Study the drawing (mm; zero at the part's minimum x, y, z) and answer. A direction names the side the tool comes from. Round coordinates to 2 decimals unless told otherwise and drop trailing zeros. Write each loop counter-clockwise with the first axis right and the second up, starting at its lowest first coordinate (ties: lowest second). Pieces come first, ordered by that corner, then holes. Notation, with made-up numbers: (33, 59.25) -> (47, 59.25) arc R19 cw to (47, 69.25) -> close; hole circle Ø3 at (29, 33). An arc over 180 degrees is marked (long way). Return JSON: item names as keys, results as strings.
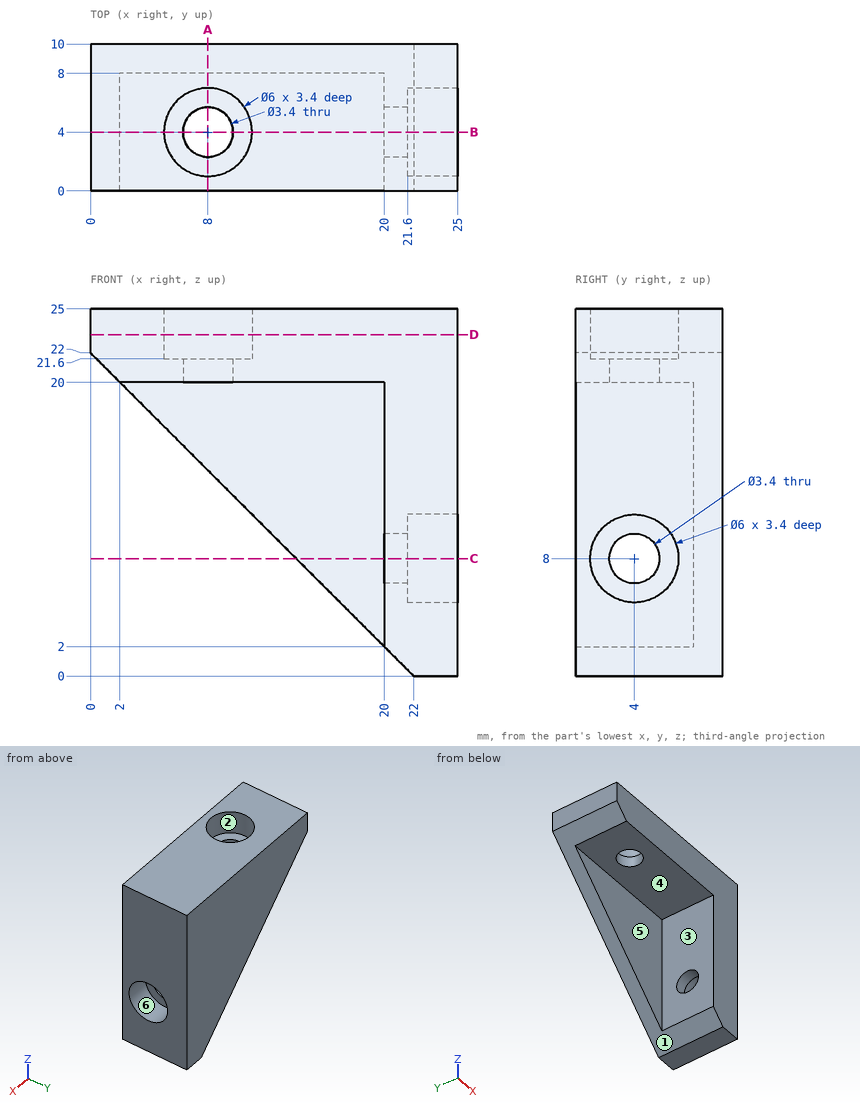
Item 1: Section D-D (z = 23.25) is taken. Give the vertices of the cut face in (x, y).
Worked answers:
{"outline": "(0, 0) -> (25, 0) -> (25, 10) -> (0, 10) -> close; hole circle Ø6 at (8, 4)"}
Item 2: Flat-ended cylindrical pins translate along their axes: pin 1 (5 mm diameter, centred on x = 8, y = 4, fed in from -Z); pin 2 (5 mm diameter, centred on x = 14, z = 3, fed in from -Y); pin 3 (6 mm diameter, centred on y = 3, z = 10.5, fed in from -X); pin 4 (1.8 mm diameter, centred on y = 4.5, z = 9.5, fed in from +X). Find the tip coordinate at first contact, or state that the pin passes through.
Worked answers:
{"pin 1": "stops at z = 20", "pin 2": "passes through", "pin 3": "stops at x = 20", "pin 4": "stops at x = 21.6"}
Item 3: Section A-A (x = 8) is taken. Give the vertices of the cut face in (y, z), then the cut area to 3 significant figures.
Worked answers:
{"outline": "(0, 20) -> (2.3, 20) -> (2.3, 21.6) -> (1, 21.6) -> (1, 25) -> (0, 25) -> close; (5.7, 20) -> (8, 20) -> (8, 14) -> (10, 14) -> (10, 25) -> (7, 25) -> (7, 21.6) -> (5.7, 21.6) -> close", "area": "36.2 mm2"}
Item 4: For a pull along Y with two mould halves and no side action, classify the marked faces 4, 5 and 6 as released by +Y, released by -Y, zero draft, split by the parting line, or undercut.
Worked answers:
{"face 4": "zero draft", "face 5": "released by -Y", "face 6": "undercut"}
Item 5: Straight lines are drawn through the part: L1, parallel to Y at x = 8, z = 22.8; L2, parallel to Y at x = 21.15, z = 8; L3, parallel to Z at x = 23.25, y = 4. For each, find the intervals that lie inside material, in ascending order. Write a range as [from, to].
Worked answers:
{"L1": "y = [0, 1], [7, 10]", "L2": "y = [0, 2.3], [5.7, 10]", "L3": "z = [0, 5], [11, 25]"}
Item 6: Section C-C (z = 8) is taken. Give the vertices of the cut face in (x, y), then the cut area to 3 significant figures.
Worked answers:
{"outline": "(14, 8) -> (20, 8) -> (20, 5.7) -> (21.6, 5.7) -> (21.6, 7) -> (25, 7) -> (25, 10) -> (14, 10) -> close; (20, 0) -> (25, 0) -> (25, 1) -> (21.6, 1) -> (21.6, 2.3) -> (20, 2.3) -> close", "area": "36.2 mm2"}
Item 7: A tool of negligible diameter and unlimited length cuts with its end or side. For the marked faces 1, 2 and 3, from which of +Z, -Z, +X, -X, +Y, -Y can it reach the whole face along a straight path? Write none if from no direction.
Worked answers:
{"face 1": "-Z, -X, +Y, -Y", "face 2": "+Z", "face 3": "-Z, -X, -Y"}
Item 8: Section B-B (y = 4) is taken. Give the vertices of the cut face in (x, z).
Worked answers:
{"outline": "(0, 22) -> (2, 20) -> (6.3, 20) -> (6.3, 21.6) -> (5, 21.6) -> (5, 25) -> (0, 25) -> close; (9.7, 20) -> (20, 20) -> (20, 9.7) -> (21.6, 9.7) -> (21.6, 11) -> (25, 11) -> (25, 25) -> (11, 25) -> (11, 21.6) -> (9.7, 21.6) -> close; (20, 2) -> (22, 0) -> (25, 0) -> (25, 5) -> (21.6, 5) -> (21.6, 6.3) -> (20, 6.3) -> close"}
